from build123d import *

# Parameters (mm, degrees)
F0_W     = 62.992
F0_H     = 15.748
F1_DEPTH = 3.20802
F2_R     = 2.4638
F3_DEPTH = 4.953
F4_T     = -1.5748
F5_R     = 3.2766
F5_R_2   = 2.4638
F6_DEPTH = 1.63322


with BuildPart() as f1:
    # F0 (on Top) → F1 (new body)
    with BuildSketch(Plane.XY):
        Rectangle(F0_W, F0_H)
    extrude(amount=F1_DEPTH)

    # F2 (on Top) → F3 (join)
    with BuildSketch(Plane.XY):
        with Locations((27.559, 3.937)):
            Circle(F2_R)
        with Locations((11.811, 3.937)):
            Circle(F2_R)
        with Locations((19.685, 3.937)):
            Circle(F2_R)
        with Locations((3.937, 3.937)):
            Circle(F2_R)
        with Locations((-3.937, 3.937)):
            Circle(F2_R)
        with Locations((-11.811, 3.937)):
            Circle(F2_R)
        with Locations((-19.685, 3.937)):
            Circle(F2_R)
        with Locations((-27.559, 3.937)):
            Circle(F2_R)
        with Locations((-27.559, -3.937)):
            Circle(F2_R)
        with Locations((-19.685, -3.937)):
            Circle(F2_R)
        with Locations((-11.811, -3.937)):
            Circle(F2_R)
        with Locations((-3.937, -3.937)):
            Circle(F2_R)
        with Locations((3.937, -3.937)):
            Circle(F2_R)
        with Locations((11.811, -3.937)):
            Circle(F2_R)
        with Locations((19.685, -3.937)):
            Circle(F2_R)
        with Locations((27.559, -3.937)):
            Circle(F2_R)
    extrude(amount=F3_DEPTH)

    # F4
    f4_openings = [f1.faces().sort_by_distance(p)[0] for p in [
        (0, 0, 0),
    ]]
    offset(amount=F4_T, openings=f4_openings, kind=Kind.INTERSECTION)

    # F5 (on face) → F6 (join)
    with BuildSketch(Plane(origin=(0, 0, 1.63322), x_dir=(1, 0, 0), z_dir=(0, 0, -1))):
        with Locations((-23.622, 0)):
            Circle(F5_R)
        with Locations((-23.622, 0)):
            Circle(F5_R_2, mode=Mode.SUBTRACT)
        with BuildLine():
            Line((-13.2842, 0), (-12.573, 0))
            ThreePointArc((-12.573, 0), (-15.748, 3.175), (-18.923, 0))
            Line((-18.923, 0), (-18.2118, 0))
            ThreePointArc((-18.2118, 0), (-15.748, 2.4638), (-13.2842, 0))
        make_face()
        with BuildLine():
            ThreePointArc((-18.923, 0), (-15.748, -3.175), (-12.573, 0))
            Line((-12.573, 0), (-13.2842, 0))
            ThreePointArc((-13.2842, 0), (-15.748, -2.4638), (-18.2118, 0))
            Line((-18.2118, 0), (-18.923, 0))
        make_face()
        with BuildLine():
            ThreePointArc((-11.049, 0), (-7.874, -3.175), (-4.699, 0))
            Line((-4.699, 0), (-5.4102, 0))
            ThreePointArc((-5.4102, 0), (-7.874, -2.4638), (-10.3378, 0))
            Line((-10.3378, 0), (-11.049, 0))
        make_face()
        with BuildLine():
            Line((-5.4102, 0), (-4.699, 0))
            ThreePointArc((-4.699, 0), (-7.874, 3.175), (-11.049, 0))
            Line((-11.049, 0), (-10.3378, 0))
            ThreePointArc((-10.3378, 0), (-7.874, 2.4638), (-5.4102, 0))
        make_face()
        with BuildLine():
            ThreePointArc((-2.4638, 0), (0, 2.4638), (2.4638, 0))
            Line((2.4638, 0), (3.175, 0))
            ThreePointArc((3.175, 0), (0, 3.175), (-3.175, 0))
            Line((-3.175, 0), (-2.4638, 0))
        make_face()
        with BuildLine():
            Line((3.175, 0), (2.4638, 0))
            ThreePointArc((2.4638, 0), (0, -2.4638), (-2.4638, 0))
            Line((-2.4638, 0), (-3.175, 0))
            ThreePointArc((-3.175, 0), (0, -3.175), (3.175, 0))
        make_face()
        with BuildLine():
            Line((5.4102, 0), (4.699, 0))
            ThreePointArc((4.699, 0), (7.874, -3.175), (11.049, 0))
            Line((11.049, 0), (10.3378, 0))
            ThreePointArc((10.3378, 0), (7.874, -2.4638), (5.4102, 0))
        make_face()
        with BuildLine():
            ThreePointArc((11.049, 0), (7.874, 3.175), (4.699, 0))
            Line((4.699, 0), (5.4102, 0))
            ThreePointArc((5.4102, 0), (7.874, 2.4638), (10.3378, 0))
            Line((10.3378, 0), (11.049, 0))
        make_face()
        with BuildLine():
            ThreePointArc((18.923, 0), (15.748, 3.175), (12.573, 0))
            Line((12.573, 0), (13.2842, 0))
            ThreePointArc((13.2842, 0), (15.748, 2.4638), (18.2118, 0))
            Line((18.2118, 0), (18.923, 0))
        make_face()
        with BuildLine():
            Line((13.2842, 0), (12.573, 0))
            ThreePointArc((12.573, 0), (15.748, -3.175), (18.923, 0))
            Line((18.923, 0), (18.2118, 0))
            ThreePointArc((18.2118, 0), (15.748, -2.4638), (13.2842, 0))
        make_face()
        with BuildLine():
            ThreePointArc((26.797, 0), (23.622, 3.175), (20.447, 0))
            ThreePointArc((20.447, 0), (23.622, -3.175), (26.797, 0))
        make_face()
        with BuildLine():
            ThreePointArc((26.0858, 0), (23.622, -2.4638), (21.1582, 0))
            ThreePointArc((21.1582, 0), (23.622, 2.4638), (26.0858, 0))
        make_face(mode=Mode.SUBTRACT)
    extrude(amount=F6_DEPTH)


solid = f1.part
Input: part model. Units: mm. Frame: model coordinates. A direction names the side the tool comes from. Coordinates: 2 decimals unless noted, no trailing zeros. Loops run counter-clockwise (first coordinate to the right, second up) from the corner with the lowest first, then second, coordinate; pieces in that order, holes last. Notation, with made-up numbers: (-36.75, 15) -> (21.25, 15) arc R9 cw to (21.25, 20) -> close; hole circle Ø6 at (36.5, 64). An arc over 180 degrees is marked (long way). One line per item, written item: value.
(1) Pin query (flat end, axial travel): pin 1 Ø2 at (y, z) = (3, 3.5) entering from -X; pin 2 Ø2.5 at (x, y) = (-8.5, -0.5) entering from -Z; pin 3 Ø1.4 at (x, y) = (27.5, 4) entering from -Z; pin 4 Ø4.5 at (x, y) = (7.874, 0) entering from +Z. Return the tip coordinate at first contact, or that it passes through.
Answer below:
pin 1: stops at x = -31.5
pin 2: stops at z = 1.63
pin 3: stops at z = 3.38
pin 4: stops at z = 3.21
(2) Cut plane A-A (x = 0). Output: boundary loops of the cut face in (y, z) (3 decimals), then the cut area to 3 significant figures.
Answer below:
outline: (-7.874, 0) -> (-6.299, 0) -> (-6.299, 1.633) -> (-3.175, 1.633) -> (-3.175, 0) -> (-2.464, 0) -> (-2.464, 1.633) -> (2.464, 1.633) -> (2.464, 0) -> (3.175, 0) -> (3.175, 1.633) -> (6.299, 1.633) -> (6.299, 0) -> (7.874, 0) -> (7.874, 3.208) -> (-7.874, 3.208) -> close
area: 32.3 mm2
(3) Draft query along Y for faces 4 (the face through (4, 4, 4.953)), 5 (the face through (17.224, -3.829, 4.068)). Return one class per face: pulls with the +Y half, pulls with the -Y half, needs draft (parallel to the pull), parting line crosses it, or undercut.
Answer below:
face 4: needs draft
face 5: undercut
(4) Set-up query: faces 1 (the face through (2.12, 5.6, 4.07)), 2 (the face through (0, 0, 1.633)), 3 (the face through (-28, 4, 4.953)). Return all of +Z, -Z, +X, -X, +Y, -Y with unobstructed straight access to the full face (end or side cutting, diameter ignored); none if empty.
Answer below:
face 1: +Z
face 2: -Z
face 3: +Z, +X, -X, +Y, -Y
(5) Ray query, line 1 along Y through (x, z) = (16, 1.4); line 2 along Y through (x, z) = (15, 0.35); line 3 along Y through (x, z) = (12, 0.7). Return the intervals inside material, ascending.
Answer below:
line 1: y = -7.87 to -6.3, -3.16 to -2.45, 2.45 to 3.16, 6.3 to 7.87
line 2: y = -7.87 to -6.3, -3.09 to -2.35, 2.35 to 3.09, 6.3 to 7.87
line 3: y = -7.87 to -6.3, 6.3 to 7.87
